```python
from build123d import *

# Parameters (mm, degrees)
F0_R     = 7.5
F0_R_2   = 4
F1_DEPTH = 24
F2_W     = 0.5
F2_H     = 1.1
F4_R     = 0.8


with BuildPart() as f1:
    # F0 (on Top) → F1 (new body)
    with BuildSketch(Plane.XY):
        Circle(F0_R)
        Circle(F0_R_2, mode=Mode.SUBTRACT)
    extrude(amount=F1_DEPTH)

    # F2 (on Front) → F3 (revolve, cut)
    with BuildSketch(Plane.XZ):
        with Locations((-7.25, 20.2)):
            Rectangle(F2_W, F2_H)
        with Locations((-7.25, 3.8)):
            Rectangle(F2_W, F2_H)
    revolve(axis=Axis((0, 0, 12), (0, 0, 1)), mode=Mode.SUBTRACT)

    # F4
    f4_edges = [f1.edges().sort_by_distance(p)[0] for p in [
        (-7.5, 0, 24),
        (-7.5, 0, 0),
    ]]
    fillet(f4_edges, radius=F4_R)


solid = f1.part
```
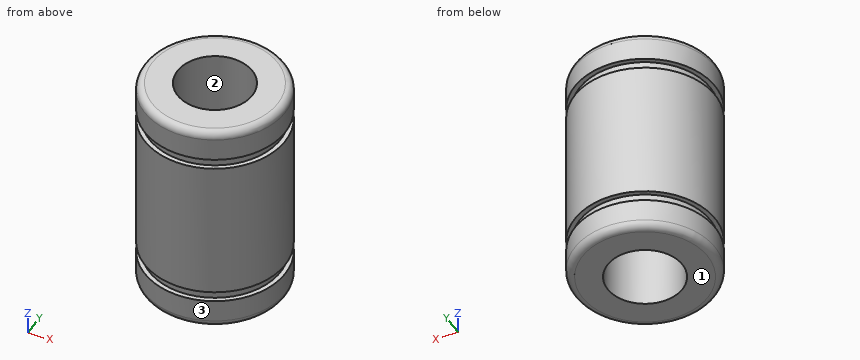
Source: CAD feature listing. Evaluate the final solid. Frame: model axes, mm. Face numbers are marked on the shaded views. Round coordinates to 2 decimals unless told otherwise and drop trailing zeros. Loops run counter-clockwise (first coordinate to the right, second up) from the corner with the lowest first, then second, coordinate; pieces in that order, holes last.
(1) Contact query for flat-ended pins moving along their axis: pin 1 Ø3 at (y, z) = (-3.5, 3.5) entering from -X; pin 2 Ø5 at (y, z) = (6, 15) entering from +X; pin 3 Ø5 at (y, z) = (-4.5, 20.5) entering from +X; pin 4 Ø6.5 at (x, y) = (0, 0) entering from +Z. Output: stop coordinate, or through.
From the geometry:
pin 1: stops at x = -7.22
pin 2: stops at x = 6.63
pin 3: stops at x = 7.22
pin 4: passes through
(2) Material intervals for probe 1 along Y at (x, z) = (0, 6.25); probe 2 along X at (y, z) = (-1, 1); probe 3 along Y at (x, z) = (-3, 2.5), sorted ascending.
From the geometry:
probe 1: y = -7.5 to -4, 4 to 7.5
probe 2: x = -7.43 to -3.87, 3.87 to 7.43
probe 3: y = -6.87 to -2.65, 2.65 to 6.87
(3) Section query A-A (y = 0). Output: boundary loops of the cut face in (x, z), and give its area (3 significant figures).
From the geometry:
outline: (-7.5, 0.8) arc R0.8 ccw to (-6.7, 0) - (-4, 0) - (-4, 24) - (-6.7, 24) arc R0.8 ccw to (-7.5, 23.2) - (-7.5, 20.75) - (-7, 20.75) - (-7, 19.65) - (-7.5, 19.65) - (-7.5, 4.35) - (-7, 4.35) - (-7, 3.25) - (-7.5, 3.25) - close; (4, 0) - (6.7, 0) arc R0.8 ccw to (7.5, 0.8) - (7.5, 3.25) - (7, 3.25) - (7, 4.35) - (7.5, 4.35) - (7.5, 19.65) - (7, 19.65) - (7, 20.75) - (7.5, 20.75) - (7.5, 23.2) arc R0.8 ccw to (6.7, 24) - (4, 24) - close
area: 165 mm2
(4) Pull-direction query (Y, two-part tool) for the marked faces 1, 2 and 3; classes: +Y half, -Y half, draft (parallel to the pull), parting line (faces both ways), or undercut.
From the geometry:
face 1: draft
face 2: undercut
face 3: parting line
(5) Section query C-C (z = 7.5). Output: boundary loops of the cut face in (x, y).
From the geometry:
outline: circle Ø15 at (0, 0); hole circle Ø8 at (0, 0)
